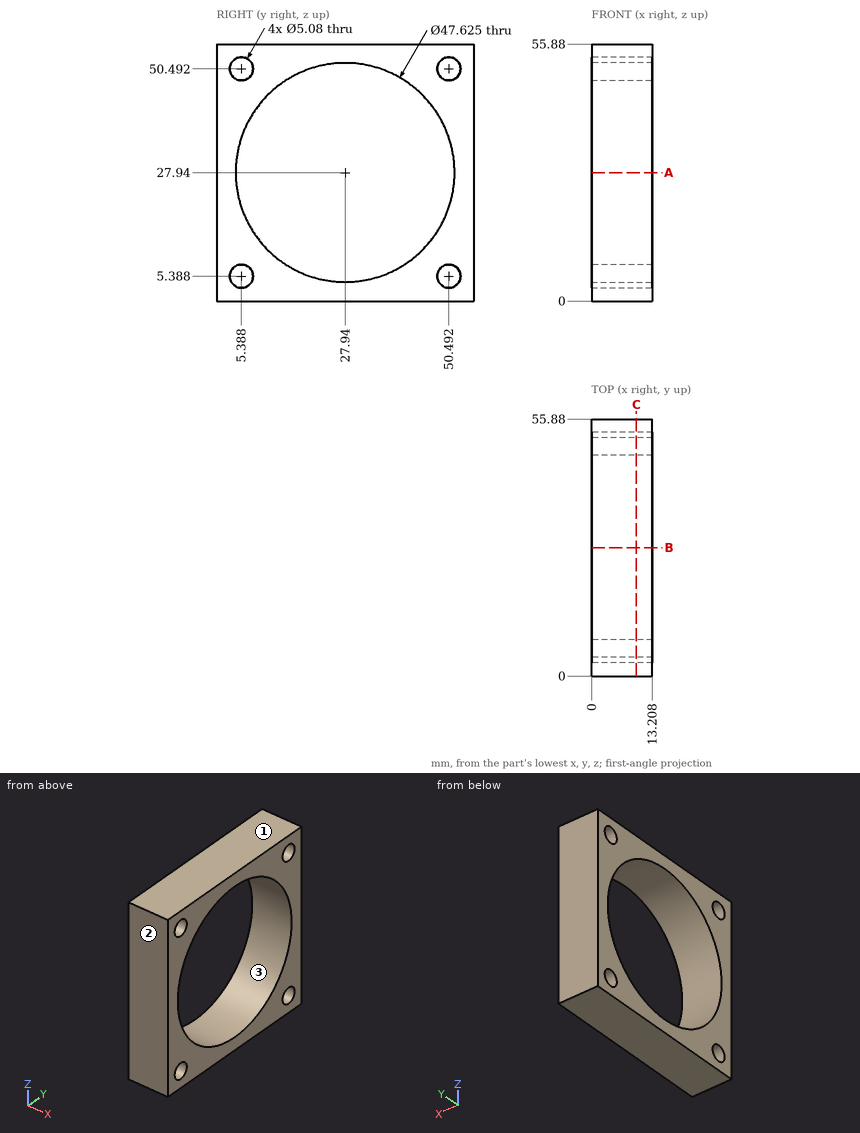
Could you check a few things on this drawing? It's one solid part, dimensions in mm from its lowest x, y, z. Give positions to 0.01 mm unless a question says otherwise; leave off trailing zeros. Loops run counter-clockwise (first coordinate to the right, second up) from the corner with the lowest first, then second, coordinate; pieces in that order, holes last. Notation, with made-up numbers: M 87.25,-10.75 L 116.25,-10.75 A24 cw 116.25,4.25 Z; hole C -38,18.5 d11. An arc over 180 degrees is marked long. One line per question, with ' | ' between items. Start each with the question number.
Q1. If I drill on line 1 (Z direction, x = 12.5, y = 28); line 2 (Z direction, x = 3.5, y = 6.5) (1 decimal), over which ranges is the centre line in solid material (lowest first)? Write a range as from..to.
Q2. If we section it at A-A (z = 27.94): Please give me the cut outline in (x, y).
Q3. If we mould it in two halves opening along Z, with no side actions, what happens to the marked faces 1, 2 and 3? For each: +Z half, -Z half, draft (parallel to the pull), parting line (faces both ways), or undercut.
Q4. If we section it at C-C (x = 9.75): Please give me the cut outline in (y, z) (1 decimal).
Computed:
1) line 1: z = 0..4.13, 51.75..55.88 | line 2: z = 0..3.1, 7.7..17.6, 38.3..48.2, 52.8..55.9
2) outline: M 0,0 L 13.21,0 L 13.21,4.13 L 0,4.13 Z; M 0,51.75 L 13.21,51.75 L 13.21,55.88 L 0,55.88 Z
3) face 1: +Z half | face 2: draft | face 3: undercut
4) outline: M 0,0 L 55.9,0 L 55.9,55.9 L 0,55.9 Z; hole C 5.4,5.4 d5.1; hole C 5.4,50.5 d5.1; hole C 27.9,27.9 d47.6; hole C 50.5,5.4 d5.1; hole C 50.5,50.5 d5.1
